Autodesk Inventor part; units mm, degrees
ref_plane "XZ Plane" through (0, 0, 0) normal (0, 1, 0) x (-1, 0, 0)
ref_plane "XY Plane" through (0, 0, 0) normal (0, 0, 1) x (1, 0, 0)
sketch "Sketch1" plane through (0, 0, 0) normal (1, 0, 0) x (0, 1, 0)
  point P0 (0, 0)
sketch "Sketch2" plane through (0, 0, 0) normal (1, 0, 0) x (0, 1, 0)
  line L0 (0, 0) -> (120, 0)
  line L1 (120, 0) -> (120, -190)
  line L2 (120, -190) -> (0, -190)
  line L3 (0, -190) -> (0, 0)
  circle A0 centre (20, -140) radius 24
  line L4 (20, -164) -> (0, -164)
  line L5 (20, -116) -> (0, -116)
  line L6 (120, -190) -> (120, -166)
  line L7 (120, -166) -> (100, -166)
  line L8 (100, -166) -> (100, -128)
  line L9 (100, -128) -> (120, -128)
  line L10 (120, -128) -> (120, -90)
  line L11 (120, -90) -> (72, -90)
  line L12 (72, -90) -> (20, -90)
  line L13 (20, -90) -> (20, 0)
  line L14 (20, 0) -> (0, 0)
  line L15 (120, 0) -> (20, 0)
  point P0 (0, -126.7335)
  point P1 (0, -153.2665)
  dimension "d0" = 190
  dimension "d1" = 120
  dimension "d4" = 48
  dimension "d5" = 20
  dimension "d6" = 50
  dimension "d7" = 24
  dimension "d8" = 20
  dimension "d9" = 38
  dimension "d10" = 38
  dimension "d11" = 48
extrude "Extrusion1" add sketch "Sketch2" against normal blind 80 contours L0 L13 L12 L11 L1 L9 L8 L7 L2 L3 L4 A0 L5 | L0 L1 L11 L12 L13 | L5 A0 L3 | A0 L3 | A0 L4 L3 | L1 L7 L8 L9 picked at (15.1537, -135.0371)
extrude "Extrusion2" cut sketch "Sketch2" against normal blind 80 contours L0 L1 L11 L12 L13 | A0 L3 | L1 L7 L8 L9 picked at (15.1537, -135.0371)
extrude "Extrusion3" cut sketch "Sketch2" against normal blind 80 contours L5 A0 L3 | A0 L4 L3
sketch "Sketch3" plane through (-80, 20, -90) normal (0, 1, 0) x (1, 0, 0)
  line L0 (80, -90) -> (0, -90)
  line L1 (40, -90) -> (40, 100)
  line L2 (80, 100) -> (0, 100)
  circle A0 centre (40, -50) radius 20
  circle A1 centre (40, -50) radius 40
  line L3 (80, -90) -> (0, -90)
  line L4 (0, -90) -> (0, 0)
  line L5 (0, -90) -> (0, 100)
  line L6 (0, -90) -> (80, -90)
  line L7 (80, 74) -> (80, 100)
  line L8 (80, -90) -> (80, 100)
  point P0 (80, -50)
  point P1 (0, -50)
  dimension "d16" = 40
  dimension "d17" = 80
  dimension "d18" = 40
extrude "Extrusion4" cut sketch "Sketch3" against normal blind 80 contours L0 A1 L8 | L0 L4 A1 | A0 L1 | L1 A0
sketch "Sketch4" plane through (-80, 120, -90) normal (0, 0, 1) x (1, 0, 0)
  line L0 (0, 0) -> (0, -120)
  line L1 (80, 0) -> (80, -100)
  line L2 (0, 0) -> (80, 0)
  line L3 (80, 0) -> (80, -120)
  line L4 (0, -120) -> (80, -120)
  line L5 (80, -120) -> (0, -120)
  line L6 (0, -120) -> (0, 0)
  line L7 (80, 0) -> (0, 0)
  line L8 (40, 0) -> (40, -120)
  line L9 (0, 0) -> (0, -48)
  line L10 (0, 0) -> (20, 0)
  line L11 (20, 0) -> (20, -48)
  line L12 (20, -48) -> (60, -48)
  line L13 (60, -48) -> (60, 0)
  dimension "d21" = 48
  dimension "d22" = 20
  dimension "d23" = 40
  dimension "d24" = 48
extrude "Extrusion5" cut sketch "Sketch4" against normal blind 100 contours L2 L8 L12 L11 | L2 L13 L12 L8
ref_plane "Work Plane1" through (-40, 72, -90) normal (1, 0, 0) x (0, 1, 0)
sketch "Sketch5" plane through (-40, 72, -90) normal (1, 0, 0) x (0, 1, 0)
  line L0 (0, 0) -> (0, -100)
  line L1 (0, 0) -> (0, 25)
  line L2 (0, 25) -> (-52, 25)
  line L3 (0, 0) -> (-52, 25)
  line L4 (-52, 50) -> (-52, 0)
  line L5 (0, 0) -> (-52, 0)
  line L6 (-52, 0) -> (-52, 25)
  point P0 (-72, 90)
  dimension "d27" = 25
  dimension "d28" = 52
extrude "Extrusion6" add sketch "Sketch5" along normal mid plane 10 contours L5 L4 L3
properties part number "2"
Geometry check sheet. Reference: the model listing, model coordinates, mm. A direction names the side the tool comes from. Give positions to 0.01 mm unless a question says otherwise; leave off trailing zeros. Order: outer loops, then holes, each group sorted by start corner. A loop starts at its lowest first (then second) coordinate and runs counter-clockwise, first axis right, second up.
1. Depth check by flat-ended pin: pin 1 (6 mm diameter, centred on x = -13, y = 30, fed in from +Z); pin 2 (7.5 mm diameter, centred on y = 55, z = -80, fed in from -X); pin 3 (12 mm diameter, centred on x = -42.5, y = 44.5, fed in from +Z); pin 4 (1.5 mm diameter, centred on y = 22.5, z = -61, fed in from +X). Enter the tip coordinate at first touch or a pass-through.
Completed:
pin 1: stops at z = -90
pin 2: stops at x = -45
pin 3: stops at z = -73.89
pin 4: passes through
2. Sectioned sample at C-C (z = -140). Record the boundary of the cut face in (x, y), then the cut area to 3 significant figures.
Completed:
outline: (-80, 44) - (0, 44) - (0, 100) - (-20, 100) - (-20, 72) - (-60, 72) - (-60, 100) - (-80, 100) - close
area: 3,360 mm2
3. Access from +Z, -Z, +X, -X, +Y, -Y to the whole of each face (thin tool, end or side, straight path). Record for faces 1 (the face through (-39, 10, -164)), 2 (the face through (-70, 110, -166)), 3 (the face through (-40, 72, -139)), 4 (the face through (-45, 34, -83)).
Completed:
face 1: +X, -X, -Y
face 2: +X, -X, +Y
face 3: +Z, -Z, +Y
face 4: +Z, -X, +Y
4. Scan lines: line 1 (Z direction, x = -40, y = 12.5); line 2 (X direction, y = 74, z = -149.5); line 3 (Y direction, x = -39.5, z = -109). Record each from-to range of solid material in increasing order.
Completed:
line 1: z = -190 to -164, -116 to -60, -20 to 0
line 2: x = -80 to -60, -20 to 0
line 3: y = 0 to 72
5. Sectioned sample at D-D (y = 109). Record the boundary of the cut face in (x, z).
Completed:
outline: (-80, -190) - (-60, -190) - (-60, -166) - (-80, -166) - close; (-80, -128) - (-60, -128) - (-60, -90) - (-80, -90) - close; (-20, -190) - (0, -190) - (0, -166) - (-20, -166) - close; (-20, -128) - (0, -128) - (0, -90) - (-20, -90) - close
6. Sectioned sample at B-B (y = 86.5). Record the boundary of the cut face in (x, z).
Completed:
outline: (-80, -190) - (-60, -190) - (-60, -90) - (-80, -90) - close; (-20, -190) - (0, -190) - (0, -90) - (-20, -90) - close
7. Draft check along Z on faces 5 (the face through (-60, 91, -139)), 6 (the face through (-10, 110, -166)), 7 (the face through (-66, 60, -90)), 8 (the face through (-39, 10, -116)). Enter one of: pulls with the +Z half, pulls with the -Z half, needs draft (parallel to the pull), parting line crosses it, or undercut.
Completed:
face 5: needs draft
face 6: undercut
face 7: pulls with the +Z half
face 8: undercut
8. Sectioned sample at A-A (x = -40). Record the boundary of the cut face in (y, z), then the cut area to 3 significant figures.
Completed:
outline: (0, -190) - (72, -190) - (72, -90) - (20, -65) - (20, -60) - (0, -60) - (0, -116) - (20, -116) arc R24 cw to (20, -164) - (0, -164) - close; (0, -20) - (20, -20) - (20, 0) - (0, 0) - close
area: 6,990 mm2
